Design review of the part built by this model. Coordinates are the model's own, in mm. Face numbers are marked on the shaded views. A direction names the side the tool comes from. Coordinates: 2 decimals unless noted, no trailing zeros. Loops run counter-clockwise (first coordinate to the right, second up) from the corner with the lowest first, then second, coordinate; pieces in that order, holes last. Notation, with made-up numbers: M 42,73.25 L 86,73.25 A21 cw 86,105.25 Z; hole C 87.25,58.25 d4. An arc over 180 degrees is marked long. Answer as a JSON object with one key per item and string values. Group by question number.
1. Consider section A-A (x = -10.5). State the section outline as (y, z) points, then the cut area to 3 significant figures.
2. Consider section D-D (x = -21). State the section outline as (y, z) points.
3. Machinability: for the marked faces 1 and 2, which of the approach directions +Z, -Z, +X, -X, +Y, -Y give a long, thin tool a straight path to every point of the face, cutting with its end or side? Answer none if there is none.
4. Draft analysis for pull direction X (two halves, no side actions). For the marked faces 3, 4 and 5, state which applies: +X half, -X half, draft (parallel to the pull), parting line (faces both ways), or undercut.
5. To check wall thickness, follow probe 1 along Z at (x, y) = (-0.5, 0.4); probe 2 along X at (y, z) = (1.25, 32); probe 3 along X at (y, z) = (0.3, 45). State the ranges of each line that lie inside material, in increasing order.
6. Consider section B-B (y = 5.5). Count the separate pieces of the cut face and the enclosed holes in it, then the cut area to 3 significant figures.
7. Insertion check: pin 1 (3 mm diameter, centred on x = -10, z = 9.5, fed in from +Y); pin 2 (3.5 mm diameter, centred on x = -0.5, z = 35, fed in from -Y). Each pin has a flat end and moves straight along its axis. Give the tip position at first contact, or say it passes through.
Autodesk Inventor part; units mm, degrees
ref_plane "Pracovní rovina1" through (-25.5, 0, 0) normal (1, 0, 0) x (0, 1, 0)
ref_plane "XZ Plane" through (0, 0, 0) normal (0, 1, 0) x (-1, 0, 0)
ref_plane "XY Plane" through (0, 0, 0) normal (0, 0, 1) x (1, 0, 0)
sketch "Náčrt1" plane through (0, 0, 0) normal (0, 0, 1) x (1, 0, 0)
  line L0 (-24.5, 0.5) -> (24.5, 0.5)
  line L1 (25, 1) -> (25, 10.5)
  line L2 (25, 10.5) -> (25.5, 10.5)
  line L3 (25.5, 10.5) -> (25.5, 0.5)
  line L4 (25, 0) -> (-25, 0)
  line L5 (-25.5, 0.5) -> (-25.5, 10.5)
  line L6 (-25.5, 10.5) -> (-25, 10.5)
  line L7 (-25, 10.5) -> (-25, 1)
  arc A0 (25, 0) -> (25.5, 0.5) centre (25, 0.5) ccw
  arc A1 (-25.5, 0.5) -> (-25, 0) centre (-25, 0.5) ccw
  arc A2 (24.5, 0.5) -> (25, 1) centre (24.5, 1) ccw
  arc A3 (-25, 1) -> (-24.5, 0.5) centre (-24.5, 1) ccw
  point P0 (0, 0)
  point P1 (-25, 0.5)
  point P2 (25, 0.5)
  point P3 (25.5, 0)
  point P4 (-25.5, 0)
  point P5 (25.5, 5.5)
  point P6 (25, 5.75)
  point P7 (-25.5, 5.5)
  point P8 (-25, 5.75)
  dimension "d0" = 51
  dimension "d1" = 25.5
  dimension "d2" = 0.5
  dimension "d3" = 0.5
  dimension "d4" = 0.5
  dimension "d7" = 10
  dimension "d34" = 0.5
  dimension "d35" = 0.5
extrude "Vysunutí1" add sketch "Náčrt1" along normal blind 50
sketch "Náčrt2" plane through (0, 0, 0) normal (0, 1, 0) x (-1, 0, 0)
  circle A0 centre (20.5, 5) radius 2
  line L0 (25.5, 0) -> (25.5, 50)
  line L1 (25, 0) -> (-25, 0)
  point P0 (0, 0)
  point P1 (-25.5, 0)
  dimension "d8" = 4
  dimension "d9" = 5
  dimension "d10" = 5
extrude "Vysunutí2" cut sketch "Náčrt2" along normal through all
pattern_linear "Obdélníkové pole1" count 5 spacing 10 along (1, 0, 0) count 5 spacing 10 along (0, 0, 1) of "Vysunutí2"
ref_plane "Pracovní rovina1" through (-25.5, 0, 0) normal (1, 0, 0) x (0, 1, 0)
sketch "Náčrt4" plane through (-25.5, 0, 0) normal (1, 0, 0) x (0, 1, 0)
  line L0 (10.5, 0) -> (0, 0)
  line L1 (0, 0) -> (0, 50)
  line L2 (2, 7) -> (8, 7)
  line L3 (2, 3) -> (8, 3)
  arc A0 (7.2361, 3) -> (7.2361, 7) centre (5, 5) ccw
  arc A1 (2.7639, 7) -> (2.7639, 3) centre (5, 5) ccw
  dimension "d21" = 5
  dimension "d22" = 5
  dimension "d23" = 6
  dimension "d24" = 4
  dimension "d25" = 2
  dimension "d26" = 6
  dimension "d27" = 3
  dimension "d28" = 3
extrude "Vysunutí3" cut sketch "Náčrt4" along normal through all
pattern_linear "Obdélníkové pole2" count 5 spacing 10 along (0, 0, 1) of "Vysunutí3"
fillet "Zaoblení1" radius 1 2 edges at (25.25, 10.5, 50) (-25.25, 10.5, 50)
fillet "Zaoblení2" radius 1 2 edges at (25.25, 10.5, 0) (-25.25, 10.5, 0)
properties part number "1035"
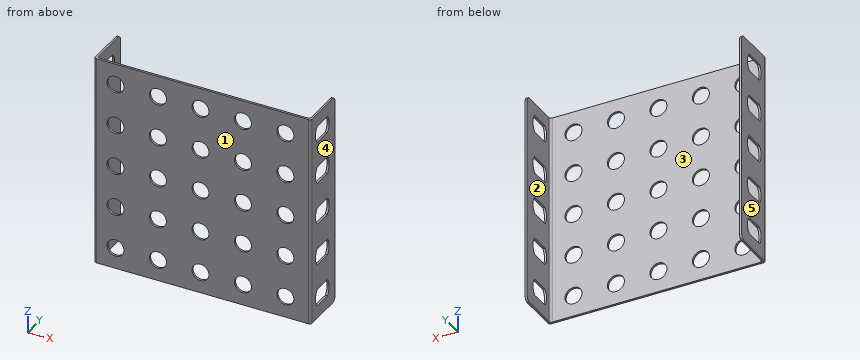
Findings below:
{
 "1": {"outline": "M 0,0 L 0.5,0 L 0.5,3 L 0,3 Z; M 0,7 L 0.5,7 L 0.5,13 L 0,13 Z; M 0,17 L 0.5,17 L 0.5,23 L 0,23 Z; M 0,27 L 0.5,27 L 0.5,33 L 0,33 Z; M 0,37 L 0.5,37 L 0.5,43 L 0,43 Z; M 0,47 L 0.5,47 L 0.5,50 L 0,50 Z", "area": "15.0 mm^2"},
 "2": {"outline": "M 0,0 L 0.5,0 L 0.5,3.06 L 0,3.06 Z; M 0,6.94 L 0.5,6.94 L 0.5,13.06 L 0,13.06 Z; M 0,16.94 L 0.5,16.94 L 0.5,23.06 L 0,23.06 Z; M 0,26.94 L 0.5,26.94 L 0.5,33.06 L 0,33.06 Z; M 0,36.94 L 0.5,36.94 L 0.5,43.06 L 0,43.06 Z; M 0,46.94 L 0.5,46.94 L 0.5,50 L 0,50 Z"},
 "3": {"face 1": "+Z, -Z, +X, -X, -Y", "face 2": "+Z, -Z, +Y"},
 "4": {"face 3": "undercut", "face 4": "+X half", "face 5": "-X half"},
 "5": {"probe 1": "z = 0 to 3, 7 to 13, 17 to 23, 27 to 33, 37 to 43, 47 to 50", "probe 2": "x = -25.5 to -25, 25 to 25.5", "probe 3": "x = -25.46 to -22.5, -18.5 to -12.5, -8.5 to -2.5, 1.5 to 7.5, 11.5 to 17.5, 21.5 to 25.46"},
 "6": {"separate pieces": "12", "enclosed holes": "0", "area": "30.0 mm^2"},
 "7": {"pin 1": "stops at y = 0.5", "pin 2": "passes through"}
}
